For this review, take the finished solid that the model builds, in its own axes (mm). A direction names the side the tool comes from. Coordinates: 2 decimals unless noted, no trailing zeros. Order: outer loops, then holes, each group sorted by start corner. A loop starts at its lowest first (then second) coordinate and runs counter-clockwise, first axis right, second up. Notation, with made-up numbers: (-16.5, 58.5) - (10.5, 58.5) arc R22 cw to (10.5, 76.5) - close; hole circle Ø1 at (61.25, 8.5). An arc over 180 degrees is marked (long way). One line per item, written item: value. Start each with the question number.
(1) Consider section C-C on x = 75. Write out the cut boundary in (y, z) (3 decimals).
(2) For faces 1 (the cylindrical face through (24.11, -97.05, 9.86)), 2 (the flat face through (40, 76, 10)), list the 3-axis set-ups (+Z, -Z, +X, -X, +Y, -Y) from which the entire face can be reached by the end or side of a thin tool; tool diameter is ignored.
(3) Consider section D-D on y = 4.5. Write out the cut boundary in (x, z).
(4) Mouldability with a two-part tool opening along Y and no side actions: class faces 3 (the flat face through (-60.26, -34.79, 9.86)), 4 (the flat face through (100, 74, 10)), 5 (the cylindrical face through (68.27, 122.19, 9.86)) as released by +Y, released by -Y, zero draft, split by the parting line, or undercut.
(5) Consider section A-A on y = 130. Write out the cut boundary in (x, z).
(6) Consider section B-B on z = 3.75. Write out the cut boundary in (x, y), then the cut area to 3 significant figures.
(7) To check wall thickness, follow line 1 along X through (y, z) = (130, 12.25); line 2 along X through (y, z) = (23.5, 12); line 3 along X through (y, z) = (-24, 10). State the ranges of each line that lie inside material, in increasing order.
(8) Clearance check with flat-ended pins moving along their axes: pin 1 (8 mm diameter, centred on x = -43, z = 3, fed in from +Y); pin 2 (4 mm diameter, centred on y = 58, z = 5, fed in from -X); pin 3 (6 mm diameter, centred on y = -53.5, z = 13, fed in from -X). State where each tip first meets the part, or that it passes through.
```python
from build123d import *

# Parameters (mm, degrees)
EXTRUDE1_DEPTH = 20
SKETCH2_R      = 8
EXTRUDE3_DEPTH = 21


with BuildPart() as part:
    # Sketch1 → Extrude1 (new body)
    with BuildSketch(Plane.XY):
        with BuildLine():
            Line((-34.641016151, -20), (-86.602540378, -50))
            ThreePointArc((-86.602540378, -50), (25.88190451, -96.592582629), (100, 0))
            Line((100, 0), (100, 150))
            Line((100, 150), (40, 150))
            Line((40, 150), (40, 0))
            ThreePointArc((40, 0), (10.352761804, -38.637033052), (-34.641016151, -20))
        make_face()
    extrude(amount=EXTRUDE1_DEPTH)

    # Sketch2 → Extrude3 (cut, through all)
    with BuildSketch(Plane.XY):
        with Locations((70, 130)):
            Circle(SKETCH2_R)
    extrude(amount=EXTRUDE3_DEPTH, mode=Mode.SUBTRACT)


solid = part.part
```
Geometry check:
1. outline: (-66.144, 0) - (123.755, 0) - (123.755, 20) - (-66.144, 20) - close; (136.245, 0) - (150, 0) - (150, 20) - (136.245, 20) - close
2. face 1: +Z, -Z, -Y
2. face 2: +Z, -Z, -X, +Y
3. outline: (40, 0) - (100, 0) - (100, 20) - (40, 20) - close
4. face 3: released by +Y
4. face 4: zero draft
4. face 5: undercut
5. outline: (40, 0) - (62, 0) - (62, 20) - (40, 20) - close; (78, 0) - (100, 0) - (100, 20) - (78, 20) - close
6. outline: (-86.6, -50) arc R100 ccw to (100, 0) - (100, 150) - (40, 150) - (40, 0) arc R40 cw to (-34.64, -20) - close; hole circle Ø16 at (70, 130)
6. area: 19,800 mm^2
7. line 1: x = 40 to 62, 78 to 100
7. line 2: x = 40 to 100
7. line 3: x = -41.57 to -32, 32 to 97.08
8. pin 1: stops at y = -22.52
8. pin 2: stops at x = 40
8. pin 3: stops at x = -86.31
